Could you check a few things on this drawing? It's one solid part, dimensions in mm from its lowest x, y, z. Give positions to 0.01 mm unless a question says otherwise; leave off trailing zeros. Loops run counter-clockwise (first coordinate to the right, second up) from the corner with the lowest first, then second, coordinate; pieces in that order, holes last. Notation, with made-up numbers: M -11,51.25 L 38,51.25 A19 cw 38,63.25 Z; hole C -11,33.5 d11. An arc over 180 degrees is marked long. Answer in a Markdown table with one row per item. Add a question column.
1. If we section it at C-C on y = 4.5: List the corners of the cut face in (x, z) for me, then the cut area to 3 significant figures.
2. If we section it at D-D on z = 67.5: List the corners of the cut face in (x, y) for me, then the cut area to 3 significant figures.
3. If we section it at A-A on z = 45: List the corners of the cut face in (x, y) for me.
4. If we section it at B-B on x = 22.5: List the corners of the cut face in (y, z) for me, then the cut area to 3 significant figures.
5. Thinking about a two-plate mould opening in Z: for the marked faces 1, 2 and 3, which applies, released by +Z, released by -Z, zero draft, split by the parting line, or undercut?
6. I need wall thicknesses on line 1 along X through (y, z) = (6.75, 22.5); line 2 along Z through (x, y) = (23, 9.75); line 3 along Z through (x, y) = (23.5, 3). Which ranges of each line are inside material? Lowest first, please. Write a range as from..to.
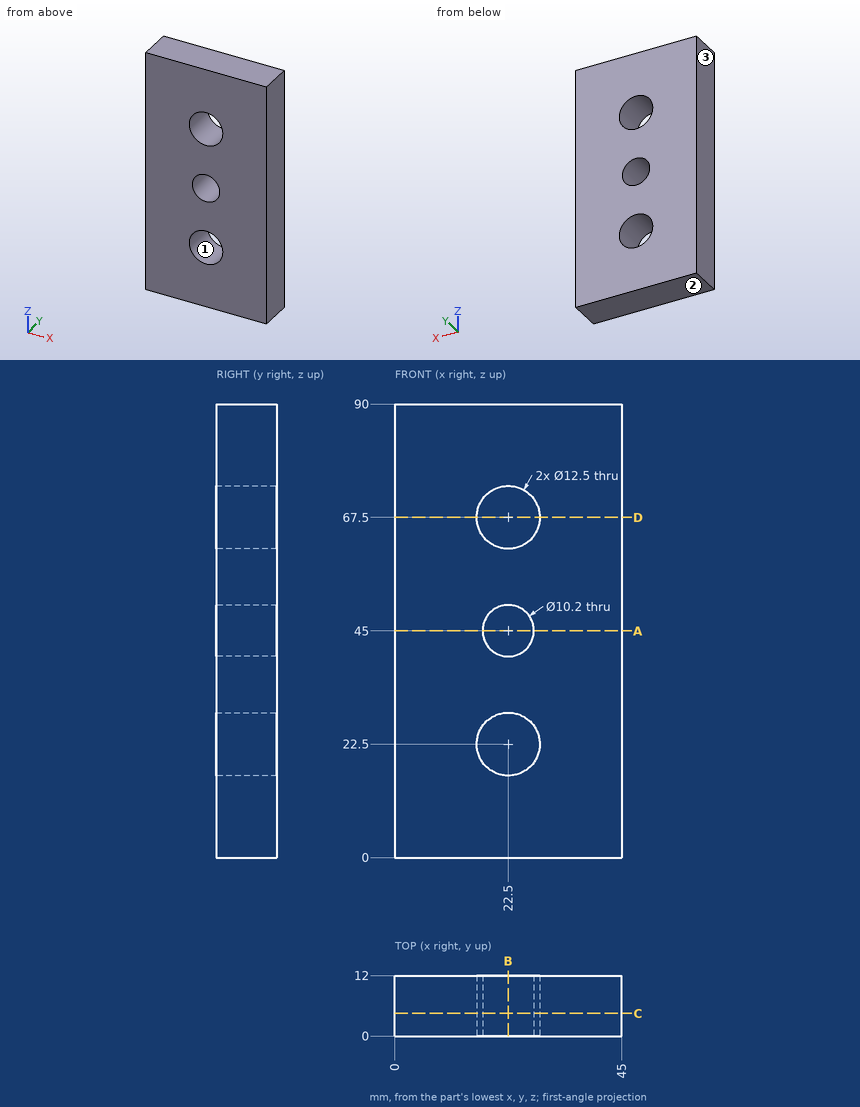
Results:
| question | item | result |
|---|---|---|
| 1 | outline | M 0,0 L 45,0 L 45,90 L 0,90 Z; hole C 22.5,22.5 d12.5; hole C 22.5,67.5 d12.5; hole C 22.5,45 d10.2 |
| 1 | area | 3,720 mm2 |
| 2 | outline | M 0,0 L 16.25,0 L 16.25,12 L 0,12 Z; M 28.75,0 L 45,0 L 45,12 L 28.75,12 Z |
| 2 | area | 390 mm2 |
| 3 | outline | M 0,0 L 17.4,0 L 17.4,12 L 0,12 Z; M 27.6,0 L 45,0 L 45,12 L 27.6,12 Z |
| 4 | outline | M 0,0 L 12,0 L 12,16.25 L 0,16.25 Z; M 0,28.75 L 12,28.75 L 12,39.9 L 0,39.9 Z; M 0,50.1 L 12,50.1 L 12,61.25 L 0,61.25 Z; M 0,73.75 L 12,73.75 L 12,90 L 0,90 Z |
| 4 | area | 658 mm2 |
| 5 | face 1 | undercut |
| 5 | face 2 | released by -Z |
| 5 | face 3 | zero draft |
| 6 | line 1 | 0..16.25, 28.75..45 |
| 6 | line 2 | 0..16.27, 28.73..39.92, 50.08..61.27, 73.73..90 |
| 6 | line 3 | 0..16.33, 28.67..40, 50..61.33, 73.67..90 |
